Check sheet for the modelled part. Datum: model origin and axes. Units: mm. A direction names the side the tool comes from. Coordinates: 2 decimals unless noted, no trailing zeros. Loops run counter-clockwise (first coordinate to the right, second up) from the corner with the lowest first, then second, coordinate; pieces in that order, holes last. Notation, with made-up numbers: (79.5, 38) -> (88.5, 38) arc R11 cw to (88.5, 53) -> close; hole circle Ø10 at (-3.5, 64.25). An arc over 180 degrees is marked (long way). Use one line per item in the form item = value.
from build123d import *

# Parameters (mm, degrees)
SKETCH1_R           = 1.5
BOSS_EXTRUDE2_DEPTH = 3


with BuildPart() as part:
    # Sketch1 → Boss-Extrude2 (new body)
    with BuildSketch(Plane.XY):
        with BuildLine():
            Line((-7.733855236, 8.750016816), (-7.733855236, -18))
            Line((-7.733855236, -18), (7.75, -18))
            Line((7.75, -18), (7.75, 9.25))
            ThreePointArc((7.75, 9.25), (-0.233977125, 16.495979574), (-7.733855236, 8.750016816))
        make_face()
        with Locations((0, -6.375)):
            Circle(SKETCH1_R, mode=Mode.SUBTRACT)
        with Locations((0, 11.125)):
            Circle(SKETCH1_R, mode=Mode.SUBTRACT)
        with BuildLine():
            ThreePointArc((10.704360482, -18), (11.593820566, -18.542987134), (11.517349886, -19.582278481))
            ThreePointArc((11.517349886, -19.582278481), (0, -25.5), (-11.517349886, -19.582278481))
            ThreePointArc((-11.517349886, -19.582278481), (-11.593820566, -18.542987134), (-10.704360482, -18))
            Line((-10.704360482, -18), (10.704360482, -18))
        make_face()
    extrude(amount=BOSS_EXTRUDE2_DEPTH)


solid = part.part
(1) Tool access check on faces 4 (the flat face through (-7.734, -4, 1)), 5 (the cylindrical face through (-0.1, 16.5, 1.5)), 6 (the flat face through (9, -18, 1)). Record the directions out of +Z, -Z, +X, -X, +Y, -Y that give a thin tool (end or side, any length) a straight path to the whole face; none if there is none.
Established:
face_4 = +Z, -Z, -X, +Y
face_5 = +Z, -Z, +Y
face_6 = +Z, -Z, +X, +Y
(2) Scan lines: line 1 along X through (y, z) = (-3, 2.05); line 2 along X through (y, z) = (10.5, 0.4); line 3 along X through (y, z) = (12.5, 2.6). Record each from-to range of solid material in increasing order.
Established:
line_1 = -7.73 to 7.75
line_2 = -7.53 to -1.36, 1.36 to 7.57
line_3 = -6.77 to -0.6, 0.6 to 6.8
(3) Section check C-C, the plane z = 1.4. Record the boundary of the cut face in (x, y) (3 decimals), plus the area to 3 significant figures.
Established:
outline = (-11.517, -19.582) arc R14.167 ccw to (11.517, -19.582) arc R1 ccw to (10.704, -18) -> (7.75, -18) -> (7.75, 9.25) arc R7.75 ccw to (-7.734, 8.75) -> (-7.734, -18) -> (-10.704, -18) arc R1 ccw to start; hole circle Ø3 at (0, -6.375); hole circle Ø3 at (0, 11.125)
area = 626 mm²
(4) Section check A-A, the plane x = 0. Record the boundary of the cut face in (y, z) (3 decimals), plus the area to 3 significant figures.
Established:
outline = (-25.5, 0) -> (-7.875, 0) -> (-7.875, 3) -> (-25.5, 3) -> close; (-4.875, 0) -> (9.625, 0) -> (9.625, 3) -> (-4.875, 3) -> close; (12.625, 0) -> (16.5, 0) -> (16.5, 3) -> (12.625, 3) -> close
area = 108 mm²
(5) Section check B-B, the plane y = -1.5. Record the boundary of the cut face in (x, z), plus the area to 3 significant figures.
Established:
outline = (-7.73, 0) -> (7.75, 0) -> (7.75, 3) -> (-7.73, 3) -> close
area = 46.5 mm²
(6) Go/stop test with a flat-tipped pin: P1, Ø0.9, axis at x = 9, z = 1, coming from the +Y side. Record where the tip stops, or that it passes through.
Established:
P1 = -18
(7) Section check D-D, the plane x = -10. Record the boundary of the cut face in (y, z), plus the area to 3 significant figures.
Established:
outline = (-21.37, 0) -> (-18, 0) -> (-18, 3) -> (-21.37, 3) -> close
area = 10.1 mm²
(8) Mould release check, pull along Y, two halves, no side actions. Record for faces 1 (the cylindrical face through (-0.33, 9.66, 1.48)), 2 (the cylindrical face through (0.2, -25.5, 1.5)), 3 (the flat face through (7.75, -5, 1)): +Y half, -Y half, draft (parallel to the pull), parting line (faces both ways), or undercut.
Established:
face_1 = undercut
face_2 = -Y half
face_3 = draft
